```python
from build123d import *

# Parameters (mm, degrees)
F0_R     = 2
F1_DEPTH = 100


with BuildPart() as f1:
    # F0 (on Top) → F1 (new body)
    with BuildSketch(Plane.XY):
        with BuildLine():
            Line((8.455436, 3), (9.5, 3))
            ThreePointArc((9.5, 3), (9.853553, 3.146447), (10, 3.5))
            Line((10, 3.5), (10, 8.5))
            ThreePointArc((10, 8.5), (9.56066, 9.56066), (8.5, 10))
            Line((8.5, 10), (3.5, 10))
            ThreePointArc((3.5, 10), (3.146447, 9.853553), (3, 9.5))
            Line((3, 9.5), (3, 8.455436))
            Line((3, 8.455436), (6, 8.455436))
            Line((6, 8.455436), (6, 6.512804))
            Line((6, 6.512804), (3.487196, 4))
            Line((3.487196, 4), (0, 4))
            Line((0, 4), (-3.487196, 4))
            Line((-3.487196, 4), (-6, 6.512804))
            Line((-6, 6.512804), (-6, 8.455436))
            Line((-6, 8.455436), (-3, 8.455436))
            Line((-3, 8.455436), (-3, 9.5))
            ThreePointArc((-3, 9.5), (-3.146447, 9.853553), (-3.5, 10))
            Line((-3.5, 10), (-8.5, 10))
            ThreePointArc((-8.5, 10), (-9.56066, 9.56066), (-10, 8.5))
            Line((-10, 8.5), (-10, 3.5))
            ThreePointArc((-10, 3.5), (-9.853553, 3.146447), (-9.5, 3))
            Line((-9.5, 3), (-8.455436, 3))
            Line((-8.455436, 3), (-8.455436, 6))
            Line((-8.455436, 6), (-6.512804, 6))
            Line((-6.512804, 6), (-4, 3.487196))
            Line((-4, 3.487196), (-4, 0))
            Line((-4, 0), (-4, -3.487196))
            Line((-4, -3.487196), (-6.512804, -6))
            Line((-6.512804, -6), (-8.455436, -6))
            Line((-8.455436, -6), (-8.455436, -3))
            Line((-8.455436, -3), (-9.5, -3))
            ThreePointArc((-9.5, -3), (-9.853553, -3.146447), (-10, -3.5))
            Line((-10, -3.5), (-10, -8.5))
            ThreePointArc((-10, -8.5), (-9.56066, -9.56066), (-8.5, -10))
            Line((-8.5, -10), (-3.5, -10))
            ThreePointArc((-3.5, -10), (-3.146447, -9.853553), (-3, -9.5))
            Line((-3, -9.5), (-3, -8.455436))
            Line((-3, -8.455436), (-6, -8.455436))
            Line((-6, -8.455436), (-6, -6.512804))
            Line((-6, -6.512804), (-3.487196, -4))
            Line((-3.487196, -4), (0, -4))
            Line((0, -4), (3.487196, -4))
            Line((3.487196, -4), (6, -6.512804))
            Line((6, -6.512804), (6, -8.455436))
            Line((6, -8.455436), (3, -8.455436))
            Line((3, -8.455436), (3, -9.5))
            ThreePointArc((3, -9.5), (3.146447, -9.853553), (3.5, -10))
            Line((3.5, -10), (8.5, -10))
            ThreePointArc((8.5, -10), (9.56066, -9.56066), (10, -8.5))
            Line((10, -8.5), (10, -3.5))
            ThreePointArc((10, -3.5), (9.853553, -3.146447), (9.5, -3))
            Line((9.5, -3), (8.455436, -3))
            Line((8.455436, -3), (8.455436, -6))
            Line((8.455436, -6), (6.512804, -6))
            Line((6.512804, -6), (4, -3.487196))
            Line((4, -3.487196), (4, 0))
            Line((4, 0), (4, 3.487196))
            Line((4, 3.487196), (6.512804, 6))
            Line((6.512804, 6), (8.455436, 6))
            Line((8.455436, 6), (8.455436, 3))
        make_face()
        Circle(F0_R, mode=Mode.SUBTRACT)
    extrude(amount=F1_DEPTH)


solid = f1.part
```
Source: CAD feature listing. Evaluate the final solid. Frame: model axes, mm. A direction names the side the tool comes from. Give positions to 0.01 mm unless a question says otherwise; leave off trailing zeros. Loops run counter-clockwise (first coordinate to the right, second up) from the corner with the lowest first, then second, coordinate; pieces in that order, holes last. Notation, with made-up numbers: (-1.5, -21.75) -> (32.5, -21.75) arc R14 ccw to (32.5, -15.75) -> close; hole circle Ø9 at (66.5, -28.5). An arc over 180 degrees is marked (long way). Put each result on its own line as item: value. Start each with the question number.
1) Material intervals for probe 1 along Y at (x, z) = (0, 32.5); probe 2 along X at (y, z) = (-5, 67), sorted ascending.
2) Cut plane A-A (x = 0). Return loops of the section in (y, z), then the cut area to 3 significant figures.
3) Contact query for flat-ended pins moving along their axis: P1, Ø3.5, axis at x = 0, z = 65.5, coming from the -Y side; P2, Ø0.8, axis at x = -9, z = 27, coming from the +Y side; P3, Ø2, axis at y = -1.5, z = 60, coming from the -X side. Output: stop coordinate, or through.
4) Reachability of faces 1 (the face through (-10, 6, 49)), 2 (the face through (4.76, 5.27, 49.3)) from +Z, -Z, +X, -X, +Y, -Y: full face, straight path, thin tool, end or side. Return the list, or none.
5) Draft query along Y for faces 3 (the face through (-0.1, 2.4, 100)), 4 (the face through (6, 7, 49)), 5 (the face through (-6, -10, 49)), 6 (the face through (-5.27, 4.76, 49.3)). Return one class per face: released by +Y, released by -Y, zero draft, split by the parting line, or undercut.
6) Cut plane B-B (x = 5). Return loops of the section in (y, z), then the cut area to 3 significant figures.
Results are:
1. probe 1: y = -4 to -2, 2 to 4
1. probe 2: x = -10 to -8.46, -5.51 to -4.49, 4.49 to 5.51, 8.46 to 10
2. outline: (-4, 0) -> (-2, 0) -> (-2, 100) -> (-4, 100) -> close; (2, 0) -> (4, 0) -> (4, 100) -> (2, 100) -> close
2. area: 400 mm2
3. P1: stops at y = -4
3. P2: stops at y = 10
3. P3: stops at x = -4
4. face 1: +Z, -Z, -X, +Y, -Y
4. face 2: +Z, -Z
5. face 3: zero draft
5. face 4: undercut
5. face 5: released by -Y
5. face 6: undercut
6. outline: (-10, 0) -> (-8.46, 0) -> (-8.46, 100) -> (-10, 100) -> close; (-5.51, 0) -> (-4.49, 0) -> (-4.49, 100) -> (-5.51, 100) -> close; (4.49, 0) -> (5.51, 0) -> (5.51, 100) -> (4.49, 100) -> close; (8.46, 0) -> (10, 0) -> (10, 100) -> (8.46, 100) -> close
6. area: 514 mm2
